from build123d import *

# Parameters (mm, degrees)
PAD_DEPTH             = 6
SKETCH003_W           = 8
SKETCH003_H           = 5
POCKET_DEPTH          = 385.012494
POLARPATTERN001_COUNT = 2
PAD001_DEPTH          = 6
POCKET001_DEPTH       = 394.833356
SKETCH006_R           = 2.15
POCKET002_DEPTH       = 396.833356
POLARPATTERN002_COUNT = 2
POLARPATTERN002_ANGLE = 60
POLARPATTERN003_COUNT = 2
POLARPATTERN004_COUNT = 2
POLARPATTERN004_ANGLE = 240
FILLET_R              = 10


with BuildPart() as part:
    # Sketch → Revolution (revolve)
    with BuildSketch(Plane.XZ):
        Polygon((55, 37), (55, 0), (22.5, 0), (22.5, -30), (20, -30), (20, 5), (52, 37), align=None)
    revolve(axis=Axis((0, 0, 0), (0, 0, 1)))

    # Sketch002 (on DatumPlane) → Pad (new body, symmetric)
    with BuildSketch(Plane.YZ):
        Polygon((53, 0.1), (62, 9.55), (62, 17.55), (53, 27), align=None)
    pad = extrude(amount=PAD_DEPTH, both=True)

    # Sketch003 → Pocket (cut, through all)
    with BuildSketch(Plane.XY):
        with Locations((0, 57.51)):
            Rectangle(SKETCH003_W, SKETCH003_H)
    pocket = extrude(amount=POCKET_DEPTH, mode=Mode.SUBTRACT)

    # PolarPattern001: Pad, Pocket ×2 about axis
    polarpattern001_axis = Axis((0, 0, 0), (0, 0, 1))
    for i in range(1, POLARPATTERN001_COUNT):
        add(pad.rotate(polarpattern001_axis, i * 360 / POLARPATTERN001_COUNT))
        add(pocket.rotate(polarpattern001_axis, i * 360 / POLARPATTERN001_COUNT), mode=Mode.SUBTRACT)

    # Sketch004 (on DatumPlane) → Pad001 (join, symmetric)
    with BuildSketch(Plane(origin=(0, 0, 0), x_dir=(0.5, 0.866025, 0), z_dir=(0.866025, -0.5, 0))):
        Polygon((52, 0), (70, 0), (70, 2), (52, 20), align=None)
    pad001 = extrude(amount=PAD001_DEPTH, both=True)

    # Sketch005 → Pocket001 (cut, through all)
    with BuildSketch(Plane.XY.offset(2)):
        Polygon((32.035898, 63.487804), (38.964102, 59.487804), (31.014102, 45.718), (24.085898, 49.718), align=None)
    pocket001 = extrude(amount=POCKET001_DEPTH, mode=Mode.SUBTRACT)

    # Sketch006 → Pocket002 (cut, through all)
    with BuildSketch(Plane.XY):
        with Locations((32.5, 56.291651)):
            Circle(SKETCH006_R)
    pocket002 = extrude(amount=POCKET002_DEPTH, mode=Mode.SUBTRACT)

    # PolarPattern002: Pad001, Pocket001, Pocket002 ×2 about axis
    polarpattern002_axis = Axis((0, 0, 0), (0, 0, 1))
    for i in range(1, POLARPATTERN002_COUNT):
        add(pad001.rotate(polarpattern002_axis, i * POLARPATTERN002_ANGLE / (POLARPATTERN002_COUNT - 1)))
        add(pocket001.rotate(polarpattern002_axis, i * POLARPATTERN002_ANGLE / (POLARPATTERN002_COUNT - 1)), mode=Mode.SUBTRACT)
        add(pocket002.rotate(polarpattern002_axis, i * POLARPATTERN002_ANGLE / (POLARPATTERN002_COUNT - 1)), mode=Mode.SUBTRACT)

    # PolarPattern003: Pad001, Pocket001, Pocket002 ×2 about axis
    polarpattern003_axis = Axis((0, 0, 0), (0, 0, 1))
    for i in range(1, POLARPATTERN003_COUNT):
        add(pad001.rotate(polarpattern003_axis, i * 360 / POLARPATTERN003_COUNT))
        add(pocket001.rotate(polarpattern003_axis, i * 360 / POLARPATTERN003_COUNT), mode=Mode.SUBTRACT)
        add(pocket002.rotate(polarpattern003_axis, i * 360 / POLARPATTERN003_COUNT), mode=Mode.SUBTRACT)

    # PolarPattern004: Pad001, Pocket001, Pocket002 ×2 about axis
    polarpattern004_axis = Axis((0, 0, 0), (0, 0, 1))
    for i in range(1, POLARPATTERN004_COUNT):
        add(pad001.rotate(polarpattern004_axis, i * POLARPATTERN004_ANGLE / (POLARPATTERN004_COUNT - 1)))
        add(pocket001.rotate(polarpattern004_axis, i * POLARPATTERN004_ANGLE / (POLARPATTERN004_COUNT - 1)), mode=Mode.SUBTRACT)
        add(pocket002.rotate(polarpattern004_axis, i * POLARPATTERN004_ANGLE / (POLARPATTERN004_COUNT - 1)), mode=Mode.SUBTRACT)

    # Fillet
    fillet_edges = [part.edges().sort_by_distance(p)[0] for p in [
        (-20, 0, 5),
    ]]
    fillet(fillet_edges, radius=FILLET_R)


solid = part.part
Design review of the part built by this model. Coordinates are the model's own, in mm. A direction names the side the tool comes from. Give positions to 0.01 mm unless a question says otherwise; leave off trailing zeros. Loops run counter-clockwise (first coordinate to the right, second up) from the corner with the lowest first, then second, coordinate; pieces in that order, holes last. Notation, with made-up numbers: (28, -33.5) - (85, -33.5) arc R36 ccw to (85, 4.5) - close; hole circle Ø1 at (-14.75, -11). An arc over 180 degrees is marked (long way). Write item = value, one per line.
1) Tool access review of faces 4 (the face through (-35.46, -49.42, 6.86)), 5 (the face through (-4, -57, 13)), 6 (the face through (-31, 54, 2)), 7 (the face through (-34.775, -51.288, 10.196)), 8 (the face through (-25.07, -55.42, 6.86)): name each direction out of +Z, -Z, +X, -X, +Y, -Y from which nothing blocks a thin tool from reaching the whole face with its end or side.
Result sheet:
face_4 = +Z, -Z, -X
face_5 = +Z, -Z
face_6 = +Z
face_7 = +Z, -X, -Y
face_8 = +Z, -Z, -Y
2) Take a section at B-B on z = -2.5. State the section outline as (x, y) points, and give its area (3 significant figures).
Result sheet:
outline = circle Ø45 at (0, 0); hole circle Ø40 at (0, 0)
area = 334 mm2
3) To check wall thickness, follow line 1 (Y direction, x = 32.5, z = 0.55); line 2 (Y direction, x = 0, z = -8.5); line 3 (Y direction, x = 32, z = 1). State the ranges of each line that lie inside material, in increasing order.
Result sheet:
line_1 = -62.07 to -58.44, -54.14 to 54.14, 58.44 to 62.07
line_2 = -22.5 to -20, 20 to 22.5
line_3 = -62.35 to -58.38, -54.2 to 54.2, 58.38 to 62.35
4) Draft analysis for pull direction X (two halves, no side actions). For faces 1 (the face through (-35.46, 49.42, 6.86)), 2 (the face through (34.775, 51.288, 10.196)), 3 (the face through (-33.136, -49.393, 6.035)), state which applies: +X half, -X half, draft (parallel to the pull), parting line (faces both ways), or undercut.
Result sheet:
face_1 = -X half
face_2 = +X half
face_3 = undercut
5) Clearance check with flat-ended pins moving along their axes: pin 1 Ø2.5 at (x, z) = (0.5, 16) entering from -Y; pin 2 Ø3 at (x, z) = (-2, 1) entering from +Y; pin 3 Ø11.5 at (x, y) = (29, 57) entering from +Z. State where each tip first meets the part, or that it passes through.
Result sheet:
pin_1 = -62
pin_2 = 55.01
pin_3 = 13.85
6) Take a section at A-A on x = 0. Count the separate pieces of the cut face and the enclosed holes in it, and give its area (3 significant figures).
Result sheet:
separate_pieces = 4
enclosed_holes = 0
area = 1,750 mm2
